from build123d import *

# Parameters (mm, degrees)
SKETCH1_W                 = 66
SKETCH1_H                 = 72
BOSS_EXTRUDE1_DEPTH       = 52
SKETCH2_W                 = 60
SKETCH2_H                 = 66
BOSS_EXTRUDE2_DEPTH       = 2.5
SKETCH3_W                 = 62
SKETCH3_H                 = 68
CUT_EXTRUDE1_DEPTH        = 13
SKETCH4_R                 = 7.9
CUT_EXTRUDE2_DEPTH        = 37.5
LPATTERN1_COUNT           = 3
LPATTERN1_PITCH           = 16.4
LPATTERN1_COUNT_DIR2      = 2
LPATTERN1_PITCH_DIR2      = 28.5
SKETCH_PATTERN1_START     = 17
SKETCH_PATTERN1_OUTLINE_R = 7.9
SKETCH_PATTERN1_DEPTH     = 37.5
FILLET1_R                 = 5
FILLET2_R                 = 2


# Read off the part's stored shape, not the designer's step: Sketch-Pattern1
with BuildPart() as part:
    # Sketch1 → Boss-Extrude1 (new body)
    with BuildSketch(Plane.XY):
        Rectangle(SKETCH1_W, SKETCH1_H)
    extrude(amount=BOSS_EXTRUDE1_DEPTH)

    # Sketch2 → Boss-Extrude2 (add)
    with BuildSketch(Plane.XY.offset(52)):
        Rectangle(SKETCH2_W, SKETCH2_H)
    extrude(amount=BOSS_EXTRUDE2_DEPTH)

    # Sketch3 → Cut-Extrude1 (cut)
    with BuildSketch(Plane(origin=(0, 0, 0), x_dir=(-1, 0, 0), z_dir=(0, 0, -1))):
        Rectangle(SKETCH3_W, SKETCH3_H)
    extrude(amount=-CUT_EXTRUDE1_DEPTH, mode=Mode.SUBTRACT)

    # Sketch4 → Cut-Extrude2 (cut)
    with BuildSketch(Plane.XY.offset(54.5)):
        with Locations((21.5, 24.5)):
            Circle(SKETCH4_R)
    cut_extrude2 = extrude(amount=-CUT_EXTRUDE2_DEPTH, mode=Mode.SUBTRACT)

    # LPattern1: Cut-Extrude2 3 × 2
    with Locations(*[(-j * LPATTERN1_PITCH_DIR2, -i * LPATTERN1_PITCH, 0) for i in range(LPATTERN1_COUNT) for j in range(LPATTERN1_COUNT_DIR2) if (i, j) != (0, 0)]):
        add(cut_extrude2, mode=Mode.SUBTRACT)

    # Sketch-Pattern1 outline → Sketch-Pattern1 (cut)
    with BuildSketch(Plane.XY.offset(SKETCH_PATTERN1_START)):
        with Locations((7.5, 16.5)):
            Circle(SKETCH_PATTERN1_OUTLINE_R)
        with Locations((-21, -16.3)):
            Circle(SKETCH_PATTERN1_OUTLINE_R)
        with Locations((-21, 16.5)):
            Circle(SKETCH_PATTERN1_OUTLINE_R)
        with Locations((7.5, 0.1)):
            Circle(SKETCH_PATTERN1_OUTLINE_R)
        with Locations((-21, 0.1)):
            Circle(SKETCH_PATTERN1_OUTLINE_R)
        with Locations((7.5, -16.3)):
            Circle(SKETCH_PATTERN1_OUTLINE_R)
        with Locations((-7, -24.7)):
            Circle(SKETCH_PATTERN1_OUTLINE_R)
        with Locations((21.5, -24.7)):
            Circle(SKETCH_PATTERN1_OUTLINE_R)
    extrude(amount=SKETCH_PATTERN1_DEPTH, mode=Mode.SUBTRACT)

    # Fillet1
    fillet1_edges = [part.edges().sort_by_distance(p)[0] for p in [
        (30, 33, 53.25),
        (-30, 33, 53.25),
        (-30, -33, 53.25),
        (30, -33, 53.25),
        (-31, -34, 6.5),
        (31, -34, 6.5),
        (31, 34, 6.5),
        (-31, 34, 6.5),
        (-33, 36, 26),
        (33, 36, 26),
        (33, -36, 26),
        (-33, -36, 26),
    ]]
    fillet(fillet1_edges, radius=FILLET1_R)

    # Fillet2
    fillet2_edges = [part.edges().sort_by_distance(p)[0] for p in [
        (0, -34, 13),
        (31, 0, 13),
        (-31, 0, 13),
        (0, 34, 13),
        (-29.535533906, 32.535533906, 13),
        (-29.535533906, -32.535533906, 13),
        (29.535533906, 32.535533906, 13),
        (29.535533906, -32.535533906, 13),
    ]]
    fillet(fillet2_edges, radius=FILLET2_R)


solid = part.part
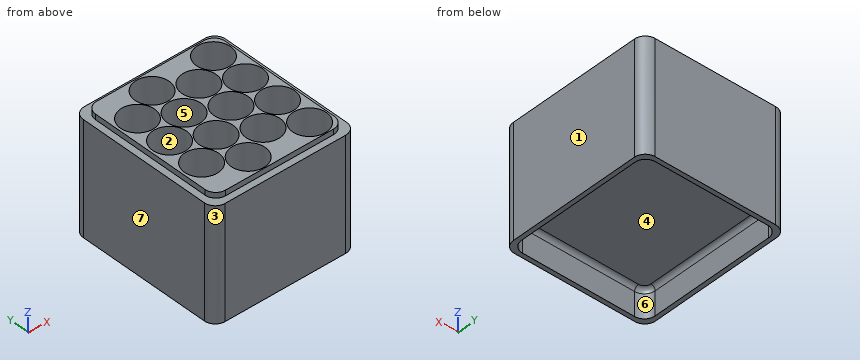
Input: part model. Units: mm. Frame: model coordinates. Face numbers are marked on the shaded views. A direction names the side the tool comes from. Coordinates: 2 decimals unless noted, no trailing zeros. Order: outer loops, then holes, each group sorted by start corner. A loop starts at its lowest first (then second) coordinate and runs counter-clockwise, first axis right, second up. Notation, with made-up numbers: M -13,58.25 L 22,58.25 A18 cw 22,72.25 Z; hole C 53,4.5 d2. An arc over 180 degrees is marked long. Answer in a Markdown table with one row per item.
(1) Section query B-B, the plane x = 7.5. Output: boundary loops of the cut face in (y, z).
Numbers:
| item | result |
|---|---|
| outline | M -36,0 L -34,0 L -34,11 A2 cw -32,13 L 32,13 A2 cw 34,11 L 34,0 L 36,0 L 36,52 L 33,52 L 33,54.5 L 24.4,54.5 L 24.4,17 L 8.6,17 L 8.6,54.5 L 8,54.5 L 8,17 L -7.8,17 L -7.8,54.5 L -8.4,54.5 L -8.4,17 L -24.2,17 L -24.2,54.5 L -33,54.5 L -33,52 L -36,52 Z |
(2) Section query A-A, the plane z = 10. Output: boundary loops of the cut face in (x, y), plus the area to 3 significant figures.
Numbers:
| item | result |
|---|---|
| outline | M -33,-31 A5 ccw -28,-36 L 28,-36 A5 ccw 33,-31 L 33,31 A5 ccw 28,36 L -28,36 A5 ccw -33,31 Z; hole M -31,-29 A5 ccw -26,-34 L 26,-34 A5 ccw 31,-29 L 31,29 A5 ccw 26,34 L -26,34 A5 ccw -31,29 Z |
| area | 536 mm^2 |
(3) Contact query for flat-ended pins moving along their axis: pin 1 Ø8 at (x, y) = (-10, 7) entering from +Z; pin 2 Ø0.8 at (y, z) = (0.5, 54) entering from -X. Output: stop coordinate, or through.
Numbers:
| item | result |
|---|---|
| pin 1 | stops at z = 17 |
| pin 2 | stops at x = -30 |
(4) Draft query along Y for the marked faces 1, 2, 3 and 4. Return one class per face: pulls with the +Y half, pulls with the -Y half, needs draft (parallel to the pull), parting line crosses it, or undercut.
Numbers:
| item | result |
|---|---|
| face 1 | needs draft |
| face 2 | undercut |
| face 3 | pulls with the -Y half |
| face 4 | undercut |
(5) Material intervals for line 1 (Y direction, x = -20.5, z = 51); line 2 (Y direction, x = -7, z = 38); line 3 (X direction, y = 8.5, z = 36), sorted ascending. Write a range as [from, to].
Numbers:
| item | result |
|---|---|
| line 1 | y = [-36, -24.18], [-8.42, -7.78], [7.98, 8.62], [24.38, 36] |
| line 2 | y = [-36, -32.6], [-16.8, -16.2], [-0.4, 0.2], [16, 16.6], [32.4, 36] |
| line 3 | x = [-33, -14.89], [0.89, 13.61], [29.39, 33] |
(6) Access query for the marked faces 5, 6 and 7. Directions: +Z, -Z, +X, -X, +Y, -Y. A direction counts if a zero-diameter tool reaches every point of the face in a straight line with its end or side. Return the directions, or none.
Numbers:
| item | result |
|---|---|
| face 5 | +Z |
| face 6 | -Z |
| face 7 | +Z, -Z, -X, +Y, -Y |
